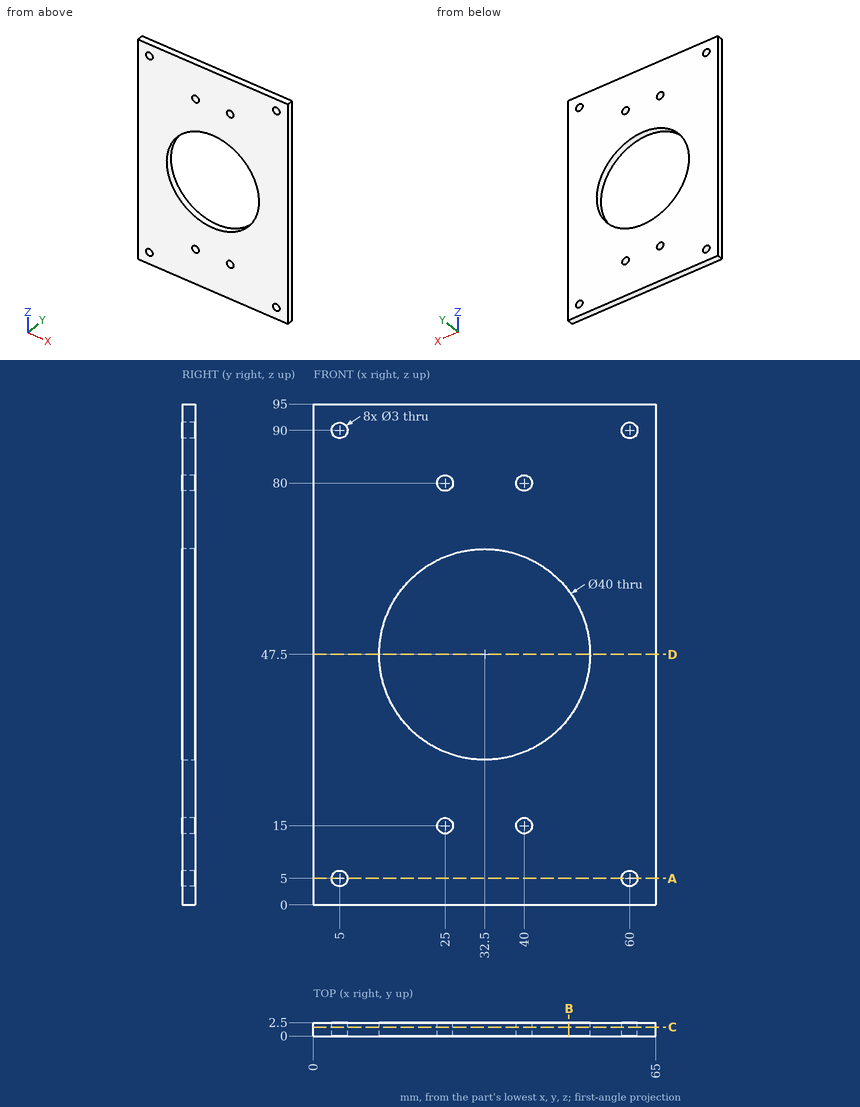
For this review, use the dimensioned drawing (mm, ordinates from the lowest corner) and the shaded views. Give positions to 0.01 mm unless a question says otherwise; leave off trailing zeros. Order: outer loops, then holes, each group sorted by start corner. A loop starts at its lowest first (then second) coordinate and runs counter-clockwise, first axis right, second up.
1) Wall thickness on line 1 (X direction, y = 1.3, z = 90); line 2 (X direction, y = 1.9, z = 80); line 3 (Z direction, x = 23, y = 1.9): over which ranges is each line inside the solid? List them lowest first.
2) Take a section at C-C (y = 1.7). State how many separate pieces and enclosed holes the cut face has, then the cut area to 3 significant figures.
3) Take a section at D-D (z = 47.5). Give the boundary of the cut face in (x, y).
4) Take a section at B-B (x = 48.5). Give the boundary of the cut face in (y, z).
5) Take a section at A-A (z = 5). Give the boundary of the cut face in (x, y), then the cut area to 4 significant figures.
Derived:
1. line 1: x = 0 to 3.5, 6.5 to 58.5, 61.5 to 65
1. line 2: x = 0 to 23.5, 26.5 to 38.5, 41.5 to 65
1. line 3: z = 0 to 29.9, 65.1 to 95
2. separate pieces: 1
2. enclosed holes: 9
2. area: 4,860 mm2
3. outline: (0, 0) - (12.5, 0) - (12.5, 2.5) - (0, 2.5) - close; (52.5, 0) - (65, 0) - (65, 2.5) - (52.5, 2.5) - close
4. outline: (0, 0) - (2.5, 0) - (2.5, 35.5) - (0, 35.5) - close; (0, 59.5) - (2.5, 59.5) - (2.5, 95) - (0, 95) - close
5. outline: (0, 0) - (3.5, 0) - (3.5, 2.5) - (0, 2.5) - close; (6.5, 0) - (58.5, 0) - (58.5, 2.5) - (6.5, 2.5) - close; (61.5, 0) - (65, 0) - (65, 2.5) - (61.5, 2.5) - close
5. area: 147.5 mm2
